The model under review builds one solid part; all positions refer to its coordinate system, in mm. Give positions to 0.01 mm unless a question says otherwise; leave off trailing zeros. Order: outer loops, then holes, each group sorted by start corner. A loop starts at its lowest first (then second) coordinate and runs counter-clockwise, first axis right, second up.
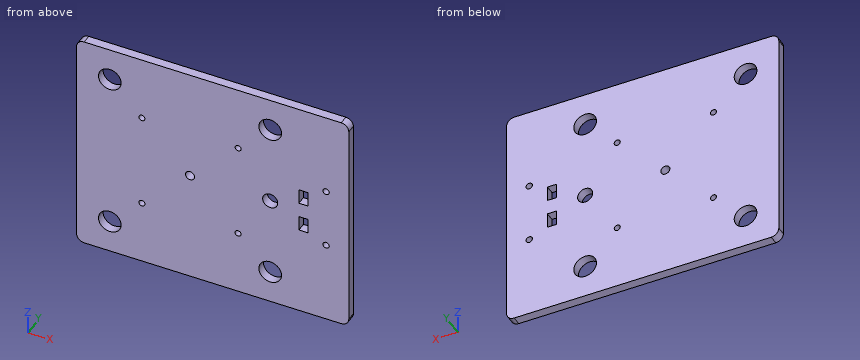
Autodesk Inventor part; units mm, degrees
ref_plane "YZ Plane" through (0, 0, 0) normal (1, 0, 0) x (0, 1, 0)
ref_plane "XZ Plane" through (0, 0, 0) normal (0, 1, 0) x (-1, 0, 0)
ref_plane "XY Plane" through (0, 0, 0) normal (0, 0, 1) x (1, 0, 0)
sketch "Sketch1" plane through (0, 0, 0) normal (0, 1, 0) x (-1, 0, 0)
  line L0 (5, 0) -> (145, 0)
  line L1 (150, -5) -> (150, -145)
  line L2 (145, -150) -> (5, -150)
  line L3 (0, -145) -> (0, -5)
  arc A0 (150, -5) -> (145, 0) centre (145, -5) ccw
  arc A1 (150, -5) -> (145, 0) centre (145, -5) ccw
  arc A2 (145, -150) -> (150, -145) centre (145, -145) ccw
  arc A3 (5, 0) -> (0, -5) centre (5, -5) ccw
  arc A4 (0, -145) -> (5, -150) centre (5, -145) ccw
  circle A5 centre (128.033, -21.967) radius 7.5
  circle A6 centre (128.033, -128.033) radius 7.5
  circle A7 centre (21.967, -128.033) radius 7.5
  circle A8 centre (21.967, -21.967) radius 7.5
  circle A9 centre (21.967, -75) radius 5
  point P0 (150, -150)
  point P1 (150, 0)
  point P2 (0, -150)
  dimension "d12" = 150
  dimension "d13" = 150
  dimension "d22" = 5
  dimension "d23" = 5
  dimension "d28" = 15
  dimension "d29" = 15
  dimension "d30" = 15
  dimension "d31" = 15
  dimension "d32" = 10
extrude "Extrusion1" add sketch "Sketch1" along normal blind 6
sketch "Sketch2" plane through (0, 6, 0) normal (0, 1, 0) x (1, 0, 0)
  arc A0 (-5, 0) -> (0, 5) centre (-5, 5) ccw
  arc A1 (-145, 150) -> (-150, 145) centre (-145, 145) ccw
  arc A2 (-150, 5) -> (-145, 0) centre (-145, 5) ccw
  circle A3 centre (-21.967, 128.033) radius 7.5
  circle A4 centre (-128.033, 21.967) radius 7.5
  circle A5 centre (-128.033, 128.033) radius 7.5
  circle A6 centre (-106.8198, 43.1802) radius 2
  circle A7 centre (-106.8198, 106.8198) radius 2
  circle A8 centre (-43.1802, 43.1802) radius 2
  circle A9 centre (-43.1802, 106.8198) radius 2
  circle A10 centre (-75, 75) radius 3
  point P0 (0, 0)
  dimension "d39" = 4
  dimension "d40" = 4
  dimension "d41" = 4
  dimension "d42" = 4
  dimension "d43" = 6
  dimension "d47" = 30
extrude "Extrusion2" cut sketch "Sketch2" against normal blind 6 contours A6 | A7 | A8 | A9 | A10
sketch "Sketch3" plane through (0, 6, 0) normal (0, 1, 0) x (1, 0, 0)
  arc A0 (-5, 0) -> (0, 5) centre (-5, 5) ccw
  line L0 (-5, 0) -> (25, 0)
  line L1 (30, 5) -> (30, 145)
  line L2 (25, 150) -> (-5, 150)
  line L3 (-5, 150) -> (-5, 0)
  arc A1 (25, 0) -> (30, 5) centre (25, 5) ccw
  arc A2 (30, 145) -> (25, 150) centre (25, 145) ccw
  point P0 (0, 0)
  point P1 (30, 150)
  point P2 (30, 0)
  dimension "d48" = 35
  dimension "d49" = 150
  dimension "d50" = 5
extrude "Extrusion3" add sketch "Sketch3" against normal blind 6
sketch "Sketch4" plane through (0, 6, 0) normal (0, 1, 0) x (1, 0, 0)
  line L0 (30, 145) -> (30, 5)
  line L1 (-3, 80) -> (3, 80)
  line L2 (3, 80) -> (3, 90)
  line L3 (3, 90) -> (-3, 90)
  line L4 (-3, 90) -> (-3, 80)
  line L5 (-3, 70) -> (3, 70)
  line L6 (3, 70) -> (3, 60)
  line L7 (3, 60) -> (-3, 60)
  line L8 (-3, 60) -> (-3, 70)
  circle A0 centre (15, 55) radius 2.1
  circle A1 centre (15, 95) radius 2.1
  line L9 (15, 55) -> (15, 75)
  line L10 (15, 75) -> (15, 95)
  point P0 (0, 0)
  dimension "d55" = 10
  dimension "d56" = 6
  dimension "d57" = 10
  dimension "d58" = 6
  dimension "d59" = 10
  dimension "d63" = 4.2
  dimension "d64" = 4.2
  dimension "d69" = 20
  dimension "d70" = 20
extrude "Extrusion4" cut sketch "Sketch4" against normal blind 6
properties part number "E_base2"
Item 1: Take a section at B-B (z = -95). Give the boundary of the cut face in (x, y), and give its area (3 significant figures).
Values found:
outline: (-150, 0) - (12.9, 0) - (12.9, 6) - (-150, 6) - close; (17.1, 0) - (30, 0) - (30, 6) - (17.1, 6) - close
area: 1,050 mm2
Item 2: Take a section at C-C (z = -123.5). Give the boundary of the cut face in (x, y), and give its area (3 significant figures).
Values found:
outline: (-150, 0) - (-134.01, 0) - (-134.01, 6) - (-150, 6) - close; (-122.06, 0) - (-27.94, 0) - (-27.94, 6) - (-122.06, 6) - close; (-15.99, 0) - (30, 0) - (30, 6) - (-15.99, 6) - close
area: 937 mm2
Item 3: Clearance check with a flat-ended pin moving along its axis: pin 1 Ø7 at (x, z) = (-75, -75) entering from +Y. State where the tip first meets the part, or that it passes through.
Values found:
pin 1: stops at y = 6
Item 4: For line 1 (X direction, y = 1.5, z = -55); line 2 (X direction, y = 2.65, z = -28.5); line 3 (Z direction, x = -72.5, y = 1.35), list the stretches that pass through material, from the lowest coordinate up.
Values found:
line 1: x = -150 to 12.9, 17.1 to 30
line 2: x = -150 to -131.72, -124.35 to -25.65, -18.28 to 30
line 3: z = -150 to -76.66, -73.34 to 0
Item 5: Take a section at D-D (x = -21). Give the boundary of the cut face in (y, z), and give its area (3 significant figures).
Values found:
outline: (0, -150) - (6, -150) - (6, -135.47) - (0, -135.47) - close; (0, -120.6) - (6, -120.6) - (6, -79.91) - (0, -79.91) - close; (0, -70.09) - (6, -70.09) - (6, -29.4) - (0, -29.4) - close; (0, -14.53) - (6, -14.53) - (6, 0) - (0, 0) - close
area: 663 mm2
Item 6: Take a section at A-A (x = 15). Give the boundary of the cut face in (y, z).
Values found:
outline: (0, -150) - (6, -150) - (6, -97.1) - (0, -97.1) - close; (0, -92.9) - (6, -92.9) - (6, -57.1) - (0, -57.1) - close; (0, -52.9) - (6, -52.9) - (6, 0) - (0, 0) - close
